from build123d import *

# Parameters (mm, degrees)
F0_W     = 40
F0_H     = 125
F1_DEPTH = 20
F2_W     = 35
F2_H     = 65
F3_DEPTH = 42.6
F5_W     = 25
F5_H     = 48
F6_DEPTH = 4
F4_R     = 1.25
F7_DEPTH = 180
F8_R     = 1.25
F9_DEPTH = 71


with BuildPart() as f1:
    # F0 (on Top) → F1 (new body)
    with BuildSketch(Plane.XY):
        Rectangle(F0_W, F0_H)
    extrude(amount=F1_DEPTH)

    # F2 (on face) → F3 (cut)
    with BuildSketch(Plane(origin=(0, 0, 0), x_dir=(1, 0, 0), z_dir=(0, 0, -1))):
        with Locations((0, -27.5)):
            Rectangle(F2_W, F2_H)
    extrude(amount=-F3_DEPTH, mode=Mode.SUBTRACT)

    # F5 (on face) → F6 (join)
    with BuildSketch(Plane.XY.offset(20)):
        with Locations((0, -33.5)):
            Rectangle(F5_W, F5_H)
    extrude(amount=F6_DEPTH)

    # F4 (on face) → F7 (cut)
    with BuildSketch(Plane.YZ.offset(20)):
        with Locations((-50.5643, 10)):
            Circle(F4_R)
    extrude(amount=-F7_DEPTH, mode=Mode.SUBTRACT)

    # F8 (on face) → F9 (cut)
    with BuildSketch(Plane.YZ.offset(20)):
        with Locations((50.281025, 10)):
            Circle(F8_R)
    extrude(amount=-F9_DEPTH, mode=Mode.SUBTRACT)


solid = f1.part
Check sheet for the modelled part. Datum: model origin and axes. Units: mm. A direction names the side the tool comes from. Round coordinates to 2 decimals unless told otherwise and drop trailing zeros. Loops run counter-clockwise (first coordinate to the right, second up) from the corner with the lowest first, then second, coordinate; pieces in that order, holes last.
1. Sectioned sample at B-B on y = 16. Record the boundary of the cut face in (x, z).
2. Gauge pin test, flat ends, axial feed: pin 1 Ø1 at (y, z) = (-15.5, 21.5) entering from +X; pin 2 Ø1.2 at (x, z) = (3, 23) entering from -Y; pin 3 Ø10 at (x, y) = (16, 11) entering from +Z. Record the tip position at first contact, or that the pin passes through.
3. Sectioned sample at A-A on x = -8. Record the boundary of the cut face in (y, z).
4. Set-up check for faces 1 (the flat face through (0, -9.5, 22)), 2 (the flat face through (12.5, -34, 22)), 3 (the flat face through (0, -57.5, 22)), 4 (the flat face through (0, 60, 10)): record each of +Z, -Z, +X, -X, +Y, -Y from which the full face is reachable in a straight line by a thin tool's end or side.
5. Sectioned sample at D-D on y = -45. Record the boundary of the cut face in (x, z).
6. Mould release check, pull along Y, two halves, no side actions. Record for faces 5 (the cylindrical face through (0.28, -49.892, 11.054)), 6 (the flat face through (0, 62.5, 10)), 7 (the cylindrical face through (18.77, 51.47, 10.38)), 8 (the flat face through (0, -27, 0)): released by +Y, released by -Y, zero draft, split by the parting line, or undercut.
7. Sectioned sample at C-C on z = 10. Record the boundary of the cut face in (x, y), and give its area (3 significant figures).
8. Scan lines: probe 1 along Y at (x, z) = (-10.5, 10.25); probe 2 along X at (y, z) = (39.5, 6.5); probe 3 along Y at (x, z) = (-6, 13.5). Record each from-to range of solid material in increasing order.
Recorded:
1. outline: (-20, 0) - (-17.5, 0) - (-17.5, 20) - (-20, 20) - close; (17.5, 0) - (20, 0) - (20, 20) - (17.5, 20) - close
2. pin 1: stops at x = 12.5
2. pin 2: stops at y = -57.5
2. pin 3: stops at z = 20
3. outline: (-62.5, 0) - (-5, 0) - (-5, 20) - (-9.5, 20) - (-9.5, 24) - (-57.5, 24) - (-57.5, 20) - (-62.5, 20) - close; (60, 0) - (62.5, 0) - (62.5, 20) - (60, 20) - close; hole circle Ø2.5 at (-50.56, 10)
4. face 1: +Z, +X, -X, +Y
4. face 2: +Z, +X, +Y, -Y
4. face 3: +Z, +X, -X, -Y
4. face 4: +Z, -Z
5. outline: (-20, 0) - (20, 0) - (20, 20) - (12.5, 20) - (12.5, 24) - (-12.5, 24) - (-12.5, 20) - (-20, 20) - close
6. face 5: undercut
6. face 6: released by +Y
6. face 7: undercut
6. face 8: zero draft
7. outline: (-20, -62.5) - (20, -62.5) - (20, -51.81) - (-20, -51.81) - close; (-20, -49.31) - (20, -49.31) - (20, 49.03) - (17.5, 49.03) - (17.5, -5) - (-17.5, -5) - (-17.5, 49.03) - (-20, 49.03) - close; (-20, 51.53) - (-17.5, 51.53) - (-17.5, 60) - (17.5, 60) - (17.5, 51.53) - (20, 51.53) - (20, 62.5) - (-20, 62.5) - close
7. area: 2,610 mm2
8. probe 1: y = -62.5 to -51.79, -49.34 to -5, 60 to 62.5
8. probe 2: x = -20 to -17.5, 17.5 to 20
8. probe 3: y = -62.5 to -5, 60 to 62.5
